Here's how the part is built. I have some questions about the finished solid (model axes, mm). A direction names the side the tool comes from. Give positions to 0.01 mm unless a question says otherwise; leave off trailing zeros. Write each loop counter-clockwise with the first axis right and the second up, starting at its lowest first coordinate (ties: lowest second). Pieces come first, ordered by that corner, then holes. Notation, with made-up numbers: (25, 26.5) - (32, 26.5) arc R15 ccw to (32, 33.5) - close; hole circle Ø4 at (76, 72.5). An arc over 180 degrees is marked (long way). Use one line per item in the form item = value. Start each with the question number.
from build123d import *

# Parameters (mm, degrees)
BOSS_EXTRUDE1_DEPTH = 2.54
BOSS_EXTRUDE2_DEPTH = 2.54
BOSS_EXTRUDE3_DEPTH = 2.54


with BuildPart() as part:
    # Sketch6 → Boss-Extrude1 (new body)
    with BuildSketch(Plane(origin=(120.788646288, 131.769432314, 69.73735745), x_dir=(-0.7587184092087563, 0.44247091722357845, 0.47808562302066715), z_dir=(-0.6295142648161258, -0.6867428343448647, -0.3634502302502976))):
        Polygon((-231.257371127, -51.055743172), (252.395306061, -422.124803926), (123.626374272, 161.135037145), align=None)
    extrude(amount=BOSS_EXTRUDE1_DEPTH)

    # Sketch7 → Boss-Extrude2 (add)
    with BuildSketch(Plane(origin=(-120.788646288, 131.769432314, 69.73735745), x_dir=(-0.7587184092087562, -0.4424709172235786, -0.4780856230206672), z_dir=(0.629514264816126, -0.6867428343448646, -0.3634502302502976))):
        Polygon((231.257371127, -51.055743172), (-252.395306061, -422.124803926), (-123.626374272, 161.135037145), align=None)
    extrude(amount=BOSS_EXTRUDE2_DEPTH)

    # Sketch9 → Boss-Extrude3 (add)
    with BuildSketch(Plane.XY):
        Polygon((0, 279.4), (304.8, 0), (-304.8, 0), align=None)
    extrude(amount=BOSS_EXTRUDE3_DEPTH)


solid = part.part
1. I want a section at C-C, the plane z = 218.5. List the corners of the cut face in (x, y) for me.
2. For P1, Ø1.5, axis at x = -56, y = 110.5, coming from the -Z side; P2, Ø1.2, axis at x = -304, z = 1, coming from the -Y side; P3, Ø1.3, axis at x = 45.5, z = 1, coming from the -Y side, each with a flat end and sliding along its axis, tell me the tip position at first contact or that it passes through.
3. I want a section at B-B, the plane x = -173.5. List the corners of the cut face in (y, z) for me.
4. Please list where these lines run through material, in increasing order: line 1 (X direction, y = 106, z = 115); line 2 (X direction, y = 22.5, z = 82.5); line 3 (Z direction, x = 3, y = 266.5).
5. For faces 1 (the face through (-149.478, 140.796, -0.455)), 2 (the face through (95.238, 83.627, 197.969)), 3 (the face through (4, 109, 0)), which set-ups out of +Z, -Z, +X, -X, +Y, -Y let a thin tool reach every point of the face, with its end or its side?
6. I want a section at A-A, the plane y = 121.5. List the corners of the cut face in (x, z) for me, then the cut area to 3 significant figures.
7. I want a section at D-D, the plane y = 33. List the corners of the cut face in (x, z) for me.
Result sheet:
q1.outline = (-178.65, 0) - (-176.52, -1.74) - (0, 160.06) - (176.52, -1.74) - (178.65, 0) - (0, 163.76) - close
q2.P1 = 0
q2.P2 = -0.75
q2.P3 = 0
q3.outline = (-1.74, 223.73) - (115.32, 2.54) - (0, 2.54) - (0, 0) - (116.66, 0) - (117.15, -0.92) - (120.36, 0) - (120.36, 2.54) - (119.01, 2.54) - (0, 227.42) - close
q4.line_1 = -122.77 to -118.73, 118.73 to 122.77
q4.line_2 = -232.62 to -228.59, 228.59 to 232.62
q4.line_3 = 0 to 2.54, 12.19 to 19.18
q5.face_1 = -Z, -X, +Y
q5.face_2 = -Y
q5.face_3 = -Z, -Y
q6.outline = (-172.25, 0) - (-168.75, -0.92) - (-168.22, 0) - (168.22, 0) - (168.75, -0.92) - (172.25, 0) - (172.25, 2.54) - (170.79, 2.54) - (0, 298.35) - (-170.79, 2.54) - (-172.25, 2.54) - close; hole (-166.75, 2.54) - (166.75, 2.54) - (0, 291.37) - close
q6.area = 3,240 mm2
q7.outline = (-268.8, 0) - (-265.3, -0.92) - (-264.77, 0) - (264.77, 0) - (265.3, -0.92) - (268.8, 0) - (268.8, 2.54) - (267.33, 2.54) - (0, 465.58) - (-267.33, 2.54) - (-268.8, 2.54) - close; hole (-263.3, 2.54) - (263.3, 2.54) - (0, 458.59) - close
